from build123d import *

# Parameters (mm, degrees)
SKETCH1_R           = 19.875
BOSS_EXTRUDE1_DEPTH = 15
SKETCH2_R           = 21
BOSS_EXTRUDE2_DEPTH = 2
SKETCH3_R           = 50
BOSS_EXTRUDE3_DEPTH = 5
CUT_EXTRUDE2_DEPTH  = 5
CUT_EXTRUDE3_DEPTH  = 2.5
SKETCH8_R           = 2.5
CUT_EXTRUDE4_DEPTH  = 20.5
BOSS_EXTRUDE4_DEPTH = 5
FILLET1_R           = 1
CHAMFER1_SIZE       = 2
SKETCH10_R          = 12.5
BOSS_EXTRUDE5_DEPTH = 5
FILLET2_R           = 1


with BuildPart() as part:
    # Sketch1 → Boss-Extrude1 (new body)
    with BuildSketch(Plane.XY):
        Circle(SKETCH1_R)
    extrude(amount=BOSS_EXTRUDE1_DEPTH)

    # Sketch2 → Boss-Extrude2 (add)
    with BuildSketch(Plane.XY.offset(15)):
        Circle(SKETCH2_R)
    extrude(amount=BOSS_EXTRUDE2_DEPTH)

    # Sketch3 → Boss-Extrude3 (add)
    with BuildSketch(Plane.XY.offset(17)):
        Circle(SKETCH3_R)
    extrude(amount=BOSS_EXTRUDE3_DEPTH)

    # Sketch4 → Cut-Extrude2 (cut)
    with BuildSketch(Plane(origin=(0, 0, 17), x_dir=(-1, 0, 0), z_dir=(0, 0, -1))):
        with BuildLine():
            ThreePointArc((-18.186533479, -10.5), (-21, 0), (-18.186533479, 10.5))
            Line((-18.186533479, 10.5), (-36.669606346, 21.484644991))
            ThreePointArc((-36.669606346, 21.484644991), (-42.499783284, 0.135723282), (-36.806079661, -21.25))
            Line((-36.806079661, -21.25), (-18.186533479, -10.5))
        make_face()
        with BuildLine():
            Line((-21.25, 36.806079661), (-10.5, 18.186533479))
            ThreePointArc((-10.5, 18.186533479), (0, 21), (10.5, 18.186533479))
            Line((10.5, 18.186533479), (21.484644991, 36.669606346))
            ThreePointArc((21.484644991, 36.669606346), (0.135723282, 42.499783284), (-21.25, 36.806079661))
        make_face()
        with BuildLine():
            Line((36.806079661, 21.25), (18.186533479, 10.5))
            ThreePointArc((18.186533479, 10.5), (20.284442352, 5.435199947), (21, 0))
            ThreePointArc((21, 0), (20.284442352, -5.435199947), (18.186533479, -10.5))
            Line((18.186533479, -10.5), (36.669606346, -21.484644991))
            ThreePointArc((36.669606346, -21.484644991), (42.499783284, -0.135723282), (36.806079661, 21.25))
        make_face()
    extrude(amount=-CUT_EXTRUDE2_DEPTH, mode=Mode.SUBTRACT)

    # Sketch5 → Cut-Extrude3 (cut)
    with BuildSketch(Plane.XY.offset(22)):
        with BuildLine():
            Line((-15, -47.696960071), (-15, -27.696960071))
            Line((-15, -27.696960071), (15, -27.696960071))
            Line((15, -27.696960071), (15, -47.696960071))
            ThreePointArc((15, -47.696960071), (0, -50), (-15, -47.696960071))
        make_face()
    extrude(amount=-CUT_EXTRUDE3_DEPTH, mode=Mode.SUBTRACT)

    # Sketch8 → Cut-Extrude4 (cut, through all)
    with BuildSketch(Plane.XY.offset(19.5)):
        with Locations((-7.5, -37.696960071)):
            Circle(SKETCH8_R)
        with Locations((7.5, -37.696960071)):
            Circle(SKETCH8_R)
    extrude(amount=-CUT_EXTRUDE4_DEPTH, mode=Mode.SUBTRACT)

    # Sketch9 → Boss-Extrude4 (add)
    with BuildSketch(Plane.XY.offset(22)):
        with BuildLine():
            Line((-36.806079661, 21.25), (-43.301270189, 25))
            ThreePointArc((-43.301270189, 25), (-49.999664861, -0.183067825), (-43.117042638, -25.316410373))
            Line((-43.117042638, -25.316410373), (-36.669606346, -21.484644991))
            ThreePointArc((-36.669606346, -21.484644991), (-42.499783284, -0.135723282), (-36.806079661, 21.25))
        make_face()
        with BuildLine():
            Line((-21.484644991, 36.669606346), (-25.316410373, 43.117042638))
            ThreePointArc((-25.316410373, 43.117042638), (-0.183067825, 49.999664861), (25, 43.301270189))
            Line((25, 43.301270189), (21.25, 36.806079661))
            ThreePointArc((21.25, 36.806079661), (-0.135723282, 42.499783284), (-21.484644991, 36.669606346))
        make_face()
        with BuildLine():
            Line((36.669606346, 21.484644991), (43.117042638, 25.316410373))
            ThreePointArc((43.117042638, 25.316410373), (49.999664861, 0.183067825), (43.301270189, -25))
            Line((43.301270189, -25), (36.806079661, -21.25))
            ThreePointArc((36.806079661, -21.25), (42.499783284, 0.135723282), (36.669606346, 21.484644991))
        make_face()
    extrude(amount=BOSS_EXTRUDE4_DEPTH)

    # Fillet1
    fillet1_edges = [part.edges().sort_by_distance(p)[0] for p in [
        (-0.183067825, 49.999664861, 27),
        (-23.400527682, 39.893324492, 27),
        (42.499783284, 0.135723282, 27),
        (40.053674925, -23.125, 27),
        (49.999664861, 0.183067825, 27),
        (39.893324492, 23.400527682, 27),
        (-42.499783284, -0.135723282, 27),
        (-40.053674925, 23.125, 27),
        (-49.999664861, -0.183067825, 27),
        (-39.893324492, -23.400527682, 27),
        (-0.135723282, 42.499783284, 27),
        (23.125, 40.053674925, 27),
    ]]
    fillet(fillet1_edges, radius=FILLET1_R)

    # Chamfer1
    chamfer1_edges = [part.edges().sort_by_distance(p)[0] for p in [
        (-19.875, 0, 0),
    ]]
    chamfer(chamfer1_edges, length=CHAMFER1_SIZE)

    # Sketch10 → Boss-Extrude5 (add)
    with BuildSketch(Plane.XY.offset(22)):
        Circle(SKETCH10_R)
    extrude(amount=BOSS_EXTRUDE5_DEPTH)

    # Fillet2
    fillet2_edges = [part.edges().sort_by_distance(p)[0] for p in [
        (-12.5, 0, 27),
    ]]
    fillet(fillet2_edges, radius=FILLET2_R)


solid = part.part
Work out the finished part from the listing and answer in its coordinate system (mm). A direction names the side the tool comes from. Coordinates: 2 decimals unless noted, no trailing zeros. Write each loop counter-clockwise with the first axis right and the second up, starting at its lowest first coordinate (ties: lowest second). Pieces come first, ordered by that corner, then holes. Notation, with made-up numbers: M 48.25,64 L 57.25,64 A26 ccw 57.25,102 Z; hole C 43.25,83 d5. An arc over 180 degrees is marked long. Use one line per item in the form item = value. Start each with the question number.
1. The mould has two halves that part along X. Classify faces 1 (the face through (-40.24, 22.9, 26.7)), 2 (the face through (0, -27.697, 21)), 3 (the face through (-23.374, 39.848, 23.972)), 4 (the face through (-45, 0, 27)): released by +X, released by -X, zero draft, split by the parting line, or undercut.
2. Straight lines are drawn through the part: probe 1 along Y at (x, z) = (-7.5, 17.7); probe 2 along X at (y, z) = (10, 23.5); probe 3 along Y at (x, z) = (19, 17.5). For each, find the intervals that lie inside material, in ascending order. Write a range as from..to.
3. Each of these flat-tipped pins is pushed along its axis until it touches: P1, Ø10, axis at y = 35.5, z = 16.5, coming from the -X side; P2, Ø18, axis at x = 4.5, y = -39.5, coming from the +Z side; P3, Ø5, axis at x = 16, z = 12.5, coming from the +Y side. Where does it stop, or does it pass through?
4. A tool of negligible diameter and unlimited length cuts with its end or side. For faces 5 (the face through (11.923, 3.755, 23.972)), 6 (the face through (-2.587, 19.706, 8.409)), 7 (the face through (39.848, 23.374, 23.972)), 8 (the face through (42.5, -0.2, 21.4)), 9 (the face through (40.15, -22.85, 26.7)), from which of +Z, -Z, +X, -X, +Y, -Y can it reach the whole face along a straight path? Write none if from no direction.
5. The part is cut by section A-A (x = -28). Give the vertices of the cut face in (y, z).
6. The part is cut by section C-C (x = 7.5). Give the number of separate pieces and of enclosed holes in the cut face, plus the area to 3 significant figures.
7. The part is cut by section B-B (z = 11.25). Give the vertices of the cut face in (x, y) (3 decimals), plus the area to 3 significant figures.
Evaluation:
q1.face_1 = undercut
q1.face_2 = undercut
q1.face_3 = released by -X
q1.face_4 = zero draft
q2.probe_1 = -49.43..-40.2, -35.2..19.62, 41.83..49.43
q2.probe_2 = -48.99..-41.31, -7.5..7.5, 41.31..48.99
q2.probe_3 = -46.25..-10.97, -8.94..8.94, 10.98..32.91, 38.02..46.25
q3.P1 = -39.6
q3.P2 = 19.5
q3.P3 = 14.59
q4.face_5 = +Z
q4.face_6 = -Z
q4.face_7 = +Z, +Y
q4.face_8 = +Z, -Z
q4.face_9 = +Z, -Y
q5.outline = M -41.42,17 L -16.33,17 L -16.33,22 L -41.42,22 Z; M 16.17,17 L 41.42,17 L 41.42,22 L 16.17,22 Z
q6.separate_pieces = 3
q6.enclosed_holes = 0
q6.area = 1,080 mm^2
q7.outline = C 0,0 d39.75
q7.area = 1,240 mm^2
